from build123d import *

# Parameters (mm, degrees)
ESBO_O1_W                                           = 68
ESBO_O1_H                                           = 20
RESSALTO_EXTRUS_O1_DEPTH                            = 8
ESCAREADO_PARA_PARAFUSO_ALLEN_SEXTAVADO_D           = 3.4
ESCAREADO_PARA_PARAFUSO_ALLEN_SEXTAVADO_CSINK_D     = 6.72
ESCAREADO_PARA_PARAFUSO_ALLEN_SEXTAVADO_CSINK_ANGLE = 90
ESBO_O4_W                                           = 4
ESBO_O4_H                                           = 20
RESSALTO_EXTRUS_O2_DEPTH                            = 24
ESBO_O5_W                                           = 45
ESBO_O5_H                                           = 20
RESSALTO_EXTRUS_O3_DEPTH                            = 8
FILETE1_R                                           = 1.6
CORTE_EXTRUS_O1_DEPTH                               = 78.768888381


with BuildPart() as part:
    # Esboço1 → Ressalto-extrusão1 (new body)
    with BuildSketch(Plane.XY):
        with Locations((34, 10)):
            Rectangle(ESBO_O1_W, ESBO_O1_H)
    extrude(amount=RESSALTO_EXTRUS_O1_DEPTH)

    # Escareado para parafuso Allen sextavado escareado de M31 (through all)
    with Locations(Plane(origin=(4, 14, 8), x_dir=(1, 0, 0), z_dir=(0, 0, 1))):
        with Locations((0, 0), (0, -8), (60, 0), (60, -8)):
            CounterSinkHole(ESCAREADO_PARA_PARAFUSO_ALLEN_SEXTAVADO_D / 2, ESCAREADO_PARA_PARAFUSO_ALLEN_SEXTAVADO_CSINK_D / 2, counter_sink_angle=ESCAREADO_PARA_PARAFUSO_ALLEN_SEXTAVADO_CSINK_ANGLE)

    # Esboço4 → Ressalto-extrusão2 (add)
    with BuildSketch(Plane.XY.offset(8)):
        with Locations((9.5, 10)):
            Rectangle(ESBO_O4_W, ESBO_O4_H)
        with Locations((58.5, 10)):
            Rectangle(ESBO_O4_W, ESBO_O4_H)
    extrude(amount=RESSALTO_EXTRUS_O2_DEPTH)

    # Esboço5 → Ressalto-extrusão3 (add)
    with BuildSketch(Plane.XY.offset(8)):
        with Locations((34, 10)):
            Rectangle(ESBO_O5_W, ESBO_O5_H)
    extrude(amount=RESSALTO_EXTRUS_O3_DEPTH)

    # Filete1
    filete1_edges = [part.edges().sort_by_distance(p)[0] for p in [
        (64.25, 20, 8),
        (64.25, 0, 8),
        (60.5, 20, 20),
        (56.5, 20, 24),
        (56.5, 0, 24),
        (60.5, 0, 20),
        (58.5, 20, 32),
        (56.5, 10, 32),
        (58.5, 0, 32),
        (60.5, 10, 32),
        (3.75, 20, 8),
        (11.5, 20, 24),
        (7.5, 20, 20),
        (7.5, 0, 20),
        (11.5, 0, 24),
        (9.5, 20, 32),
        (7.5, 10, 32),
        (9.5, 0, 32),
        (11.5, 10, 32),
        (34, 20, 16),
        (34, 0, 16),
        (0, 20, 4),
        (68, 20, 4),
        (68, 0, 4),
        (0, 0, 4),
        (3.75, 0, 8),
    ]]
    fillet(filete1_edges, radius=FILETE1_R)

    # Esboço6 → Corte-extrusão1 (cut, through all)
    with BuildSketch(Plane.XZ):
        with BuildLine():
            Line((17, 6.4), (17, 7.4))
            ThreePointArc((17, 7.4), (18.464466094, 10.935533906), (22, 12.4))
            Line((22, 12.4), (46, 12.4))
            ThreePointArc((46, 12.4), (49.535533906, 10.935533906), (51, 7.4))
            Line((51, 7.4), (51, 6.4))
            Line((51, 6.4), (51, 0))
            Line((51, 0), (17, 0))
            Line((17, 0), (17, 6.4))
        make_face()
    extrude(amount=-CORTE_EXTRUS_O1_DEPTH, mode=Mode.SUBTRACT)


solid = part.part
The model under review builds one solid part; all positions refer to its coordinate system, in mm. A direction names the side the tool comes from. Give positions to 0.01 mm unless a question says otherwise; leave off trailing zeros. Loops run counter-clockwise (first coordinate to the right, second up) from the corner with the lowest first, then second, coordinate; pieces in that order, holes last. Notation, with made-up numbers: (43.25, 53.25) -> (51.25, 53.25) arc R4 cw to (51.25, 59.25) -> close; hole circle Ø3 at (78.25, -11.5). An arc over 180 degrees is marked (long way). Put each result on its own line as item: value. Start each with the question number.
1. Wall thickness on probe 1 along Y at (x, z) = (4, 3.5); probe 2 along X at (y, z) = (6, 1.5); probe 3 along X at (y, z) = (14.5, 20): over which ranges is each line inside the solid? List them lowest first.
2. We need section D-D on z = 19. State the section outline as (x, y) points, then the cut area to 3 significant figures.
3. Mouldability with a two-part tool opening along X and no side actions: class faces 1 (the face through (9.51, 0.46, 31.52)), 2 (the face through (7.5, 10, 19)), 3 (the face through (56.5, 10, 23)) as released by +X, released by -X, zero draft, split by the parting line, or undercut.
4. We need section A-A on z = 4. State the section outline as (x, y) points.
5. We need section B-B on x = 64. State the section outline as (y, z) points.
6. Clearance check with flat-ended pins moving along their axes: P1, Ø2.5, axis at x = 64, y = 14, coming from the +Z side; P2, Ø1, axis at x = 24.5, y = 17.5, coming from the +Z side; P3, Ø8, axis at y = 10, z = 24.5, coming from the -X side; P4, Ø4, axis at x = 4, y = 14, coming from the +Z side. State where each tip first meets the part, or that it passes through.
7. We need section C-C on y = 6. State how many separate pieces and enclosed holes the cut face has, then the cut area to 3 significant figures.
8. For faces 4 (the face through (49.5, 9.86, 10.97)), 5 (the face through (4.61, 0.46, 7.52)), 6 (the face through (60.5, 10, 19)), list the 3-axis set-ups (+Z, -Z, +X, -X, +Y, -Y) from which the entire face can be reached by the end or side of a thin tool; tool diameter is ignored.
Determined:
1. probe 1: 0 to 4.3, 7.7 to 12.3, 15.7 to 20
1. probe 2: 0 to 2.3, 5.7 to 17, 51 to 62.3, 65.7 to 68
1. probe 3: 7.5 to 11.5, 56.5 to 60.5
2. outline: (7.5, 1.6) arc R1.6 ccw to (9.1, 0) -> (9.9, 0) arc R1.6 ccw to (11.5, 1.6) -> (11.5, 18.4) arc R1.6 ccw to (9.9, 20) -> (9.1, 20) arc R1.6 ccw to (7.5, 18.4) -> close; (56.5, 1.6) arc R1.6 ccw to (58.1, 0) -> (58.9, 0) arc R1.6 ccw to (60.5, 1.6) -> (60.5, 18.4) arc R1.6 ccw to (58.9, 20) -> (58.1, 20) arc R1.6 ccw to (56.5, 18.4) -> close
2. area: 156 mm^2
3. face 1: zero draft
3. face 2: released by -X
3. face 3: undercut
4. outline: (0, 1.6) arc R1.6 ccw to (1.6, 0) -> (17, 0) -> (17, 20) -> (1.6, 20) arc R1.6 ccw to (0, 18.4) -> close; (51, 0) -> (66.4, 0) arc R1.6 ccw to (68, 1.6) -> (68, 18.4) arc R1.6 ccw to (66.4, 20) -> (51, 20) -> close; hole circle Ø3.4 at (4, 6); hole circle Ø3.4 at (4, 14); hole circle Ø3.4 at (64, 6); hole circle Ø3.4 at (64, 14)
5. outline: (0, 0) -> (4.3, 0) -> (4.3, 6.34) -> (2.64, 8) -> (1.6, 8) arc R1.6 ccw to (0, 6.4) -> close; (7.7, 0) -> (12.3, 0) -> (12.3, 6.34) -> (10.64, 8) -> (9.36, 8) -> (7.7, 6.34) -> close; (15.7, 0) -> (20, 0) -> (20, 6.4) arc R1.6 ccw to (18.4, 8) -> (17.36, 8) -> (15.7, 6.34) -> close
6. P1: through
6. P2: z = 16
6. P3: x = 7.5
6. P4: z = 6.64
7. separate pieces: 3
7. enclosed holes: 0
7. area: 623 mm^2
8. face 4: -Z, +Y, -Y
8. face 5: +Z, -X, -Y
8. face 6: +Z, +X, +Y, -Y
